Can you work these out from the model? Positions are in its coordinate system, mm. Coordinates: 2 decimals unless noted, no trailing zeros. Write each loop counter-clockwise with the first axis right and the second up, starting at its lowest first coordinate (ties: lowest second). Pieces come first, ordered by that corner, then holes.
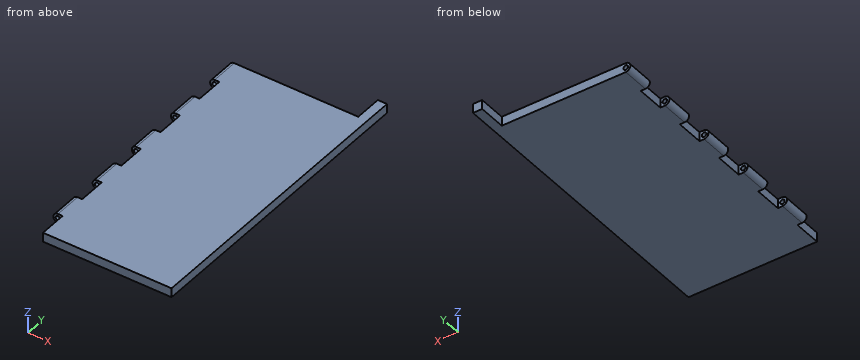
```python
from build123d import *

# Parameters (mm, degrees)
BOSS_EXTRUDE1_DEPTH = 10
SKETCH2_W           = 10
SKETCH2_H           = 30
CUT_EXTRUDE1_DEPTH  = 363.629287289
SKETCH3_R           = 2.5
CUT_EXTRUDE2_DEPTH  = 336.559234711
FILLET3_RADIUS      = 5
FILLET3_LENGTH      = 30
FILLET4_RADIUS      = 5
FILLET4_LENGTH      = 30
FILLET5_RADIUS      = 5
FILLET5_LENGTH      = 30
FILLET6_RADIUS      = 5
FILLET6_LENGTH      = 30
FILLET7_RADIUS      = 5
FILLET7_LENGTH      = 30


with BuildPart() as part:
    # Sketch1 → Boss-Extrude1 (new body)
    with BuildSketch(Plane.XY):
        Polygon((0, 0), (150, 0), (150, 206.30867798), (150, 330), (140, 330), (140, 300), (0, 300), align=None)
    extrude(amount=BOSS_EXTRUDE1_DEPTH)

    # Sketch2 → Cut-Extrude1 (cut, through all)
    with BuildSketch(Plane.XY.offset(10)):
        with Locations((5, 75)):
            Rectangle(SKETCH2_W, SKETCH2_H)
        with Locations((5, 15)):
            Rectangle(SKETCH2_W, SKETCH2_H)
        with Locations((5, 135)):
            Rectangle(SKETCH2_W, SKETCH2_H)
        with Locations((5, 195)):
            Rectangle(SKETCH2_W, SKETCH2_H)
        with Locations((5, 255)):
            Rectangle(SKETCH2_W, SKETCH2_H)
    extrude(amount=-CUT_EXTRUDE1_DEPTH, mode=Mode.SUBTRACT)

    # Sketch3 → Cut-Extrude2 (cut, through all)
    with BuildSketch(Plane(origin=(0, 300, 0), x_dir=(1, 0, 0), z_dir=(0, 1, 0))):
        with Locations(Location((5, -5, 0), (0, 0, 270))):
            Circle(SKETCH3_R)
    extrude(amount=-CUT_EXTRUDE2_DEPTH, mode=Mode.SUBTRACT)

    # Fillet3: full round fillet: the end face becomes a half cylinder, R = half its width
    fillet3_face = Plane((0, 285, 5), x_dir=(0, -1, 0), z_dir=(-1, 0, 0))  # on the end face: x along it, z out of the body
    fillet3_slab = fillet3_face.offset(-FILLET3_RADIUS / 2) * Box(FILLET3_LENGTH, 2 * FILLET3_RADIUS, FILLET3_RADIUS, mode=Mode.PRIVATE)  # the body's end, R deep
    fillet3_round = Plane((5, 285, 5), x_dir=(-1, 0, 0), z_dir=(0, -1, 0)) * Cylinder(FILLET3_RADIUS, FILLET3_LENGTH, mode=Mode.PRIVATE)  # its axis R under the face
    add(fillet3_slab - fillet3_round, mode=Mode.SUBTRACT)

    # Fillet4: full round fillet: the end face becomes a half cylinder, R = half its width
    fillet4_face = Plane((0, 225, 5), x_dir=(0, -1, 0), z_dir=(-1, 0, 0))  # on the end face: x along it, z out of the body
    fillet4_slab = fillet4_face.offset(-FILLET4_RADIUS / 2) * Box(FILLET4_LENGTH, 2 * FILLET4_RADIUS, FILLET4_RADIUS, mode=Mode.PRIVATE)  # the body's end, R deep
    fillet4_round = Plane((5, 225, 5), x_dir=(-1, 0, 0), z_dir=(0, -1, 0)) * Cylinder(FILLET4_RADIUS, FILLET4_LENGTH, mode=Mode.PRIVATE)  # its axis R under the face
    add(fillet4_slab - fillet4_round, mode=Mode.SUBTRACT)

    # Fillet5: full round fillet: the end face becomes a half cylinder, R = half its width
    fillet5_face = Plane((0, 165, 5), x_dir=(0, -1, 0), z_dir=(-1, 0, 0))  # on the end face: x along it, z out of the body
    fillet5_slab = fillet5_face.offset(-FILLET5_RADIUS / 2) * Box(FILLET5_LENGTH, 2 * FILLET5_RADIUS, FILLET5_RADIUS, mode=Mode.PRIVATE)  # the body's end, R deep
    fillet5_round = Plane((5, 165, 5), x_dir=(-1, 0, 0), z_dir=(0, -1, 0)) * Cylinder(FILLET5_RADIUS, FILLET5_LENGTH, mode=Mode.PRIVATE)  # its axis R under the face
    add(fillet5_slab - fillet5_round, mode=Mode.SUBTRACT)

    # Fillet6: full round fillet: the end face becomes a half cylinder, R = half its width
    fillet6_face = Plane((0, 105, 5), x_dir=(0, -1, 0), z_dir=(-1, 0, 0))  # on the end face: x along it, z out of the body
    fillet6_slab = fillet6_face.offset(-FILLET6_RADIUS / 2) * Box(FILLET6_LENGTH, 2 * FILLET6_RADIUS, FILLET6_RADIUS, mode=Mode.PRIVATE)  # the body's end, R deep
    fillet6_round = Plane((5, 105, 5), x_dir=(-1, 0, 0), z_dir=(0, -1, 0)) * Cylinder(FILLET6_RADIUS, FILLET6_LENGTH, mode=Mode.PRIVATE)  # its axis R under the face
    add(fillet6_slab - fillet6_round, mode=Mode.SUBTRACT)

    # Fillet7: full round fillet: the end face becomes a half cylinder, R = half its width
    fillet7_face = Plane((0, 45, 5), x_dir=(0, -1, 0), z_dir=(-1, 0, 0))  # on the end face: x along it, z out of the body
    fillet7_slab = fillet7_face.offset(-FILLET7_RADIUS / 2) * Box(FILLET7_LENGTH, 2 * FILLET7_RADIUS, FILLET7_RADIUS, mode=Mode.PRIVATE)  # the body's end, R deep
    fillet7_round = Plane((5, 45, 5), x_dir=(-1, 0, 0), z_dir=(0, -1, 0)) * Cylinder(FILLET7_RADIUS, FILLET7_LENGTH, mode=Mode.PRIVATE)  # its axis R under the face
    add(fillet7_slab - fillet7_round, mode=Mode.SUBTRACT)


solid = part.part
```
1. If we section it at B-B, the plane z = 5: Count the separate pieces of the cut face and the enclosed holes in it, plus the area to 4 significant figures.
2. If I drill on L1, parallel to X at y = 288.75, z = 5; L2, parallel to Y at x = 118.5, z = 4.5; L3, parallel to X at y = 196.5, z = 4.5, over which ranges is the centre line in solid material (lowest first)?
3. If we section it at A-A, the plane y = 295.5: List the corners of the cut face in (x, z) for me.
4. If we section it at D-D, the plane y = 259: List the corners of the cut face in (x, z) for me.
5. I'm going to push flat-ended pins straight in: P1, Ø2, axis at x = 65.5, z = 5.5, coming from the -Y side; P2, Ø4, axis at x = 5, z = 5, coming from the +Y side; P3, Ø3, axis at x = 56.5, z = 7.5, coming from the +Y side; P4, Ø5, axis at x = 5.5, z = 5.5, coming from the -Y side. Where does each tip first touch, or does it pass through?
6. If we section it at C-C, the plane x = 16: List the corners of the cut face in (y, z) for me, plus the area to 3 significant figures.
Answers:
1. separate pieces: 6
1. enclosed holes: 0
1. area: 43,050 mm2
2. L1: x = 0 to 2.5, 7.5 to 150
2. L2: y = 0 to 300
2. L3: x = 10 to 150
3. outline: (5, 0) - (150, 0) - (150, 10) - (5, 10) arc R5 ccw to start; hole circle Ø5 at (5, 5)
4. outline: (10, 0) - (150, 0) - (150, 10) - (10, 10) - close
5. P1: stops at y = 0
5. P2: passes through
5. P3: stops at y = 300
5. P4: stops at y = 30
6. outline: (0, 0) - (300, 0) - (300, 10) - (0, 10) - close
6. area: 3,000 mm2
